```python
from build123d import *

# Parameters (mm, degrees)
SKETCH2_W           = 102
SKETCH2_H           = 50
BOSS_EXTRUDE2_DEPTH = 2
SKETCH1_W           = 98
SKETCH1_H           = 46
BOSS_EXTRUDE1_DEPTH = 2
FILLET1_R           = 2
CUT_EXTRUDE1_DEPTH  = 1.6
CUT_EXTRUDE2_DEPTH  = 4
SKETCH5_OUTSIDE_W   = 126.722
SKETCH5_OUTSIDE_H   = 74.722
SKETCH5_OUTSIDE_W_2 = 95
SKETCH5_OUTSIDE_H_2 = 44
CUT_EXTRUDE3_DEPTH  = 10
SKETCH6_R           = 0.25
CUT_EXTRUDE4_DEPTH  = 10
SKETCH7_R           = 1.7
CUT_EXTRUDE5_DEPTH  = 10


with BuildPart() as part:
    # Sketch2 → Boss-Extrude2 (new body)
    with BuildSketch(Plane(origin=(0, 0, 0), x_dir=(1, 0, 0), z_dir=(0, 1, 0))):
        Rectangle(SKETCH2_W, SKETCH2_H)
    extrude(amount=BOSS_EXTRUDE2_DEPTH)

    # Sketch1 → Boss-Extrude1 (add)
    with BuildSketch(Plane(origin=(0, 0, 0), x_dir=(1, 0, 0), z_dir=(0, 1, 0))):
        Rectangle(SKETCH1_W, SKETCH1_H)
    extrude(amount=BOSS_EXTRUDE1_DEPTH)

    # Fillet1
    fillet1_edges = [part.edges().sort_by_distance(p)[0] for p in [
        (51, 1, 25),
        (-51, 1, 25),
        (-51, 1, -25),
        (51, 1, -25),
    ]]
    fillet(fillet1_edges, radius=FILLET1_R)

    # Sketch3 → Cut-Extrude1 (cut)
    with BuildSketch(Plane(origin=(0, 2, 0), x_dir=(1, 0, 0), z_dir=(0, 1, 0))):
        with BuildLine():
            ThreePointArc((-45.25, 19.75), (-46.957106781, 20.457106781), (-46.25, 18.75))
            Line((-46.25, 18.75), (-46.25, 19.75))
            Line((-46.25, 19.75), (-45.25, 19.75))
        make_face()
        with BuildLine():
            Line((-46.25, 19.75), (-46.25, 18.75))
            ThreePointArc((-46.25, 18.75), (-45.542893219, 19.042893219), (-45.25, 19.75))
            Line((-45.25, 19.75), (-46.25, 19.75))
        make_face()
        with BuildLine():
            Line((-46.25, -18.75), (-46.25, -19.75))
            Line((-46.25, -19.75), (-45.25, -19.75))
            ThreePointArc((-45.25, -19.75), (-45.542893219, -19.042893219), (-46.25, -18.75))
        make_face()
        with BuildLine():
            Line((-45.25, -19.75), (-46.25, -19.75))
            Line((-46.25, -19.75), (-46.25, -18.75))
            ThreePointArc((-46.25, -18.75), (-46.957106781, -20.457106781), (-45.25, -19.75))
        make_face()
        with BuildLine():
            ThreePointArc((46.25, -18.75), (45.542893219, -19.042893219), (45.25, -19.75))
            Line((45.25, -19.75), (46.25, -19.75))
            Line((46.25, -19.75), (46.25, -18.75))
        make_face()
        with BuildLine():
            Line((46.25, -19.75), (45.25, -19.75))
            ThreePointArc((45.25, -19.75), (46.25, -20.75), (47.25, -19.75))
            ThreePointArc((47.25, -19.75), (46.957106781, -19.042893219), (46.25, -18.75))
            Line((46.25, -18.75), (46.25, -19.75))
        make_face()
        with BuildLine():
            ThreePointArc((45.25, 19.75), (45.542893219, 19.042893219), (46.25, 18.75))
            Line((46.25, 18.75), (46.25, 19.75))
            Line((46.25, 19.75), (45.25, 19.75))
        make_face()
        with BuildLine():
            Line((46.25, 19.75), (46.25, 18.75))
            ThreePointArc((46.25, 18.75), (46.957106781, 19.042893219), (47.25, 19.75))
            ThreePointArc((47.25, 19.75), (46.25, 20.75), (45.25, 19.75))
            Line((45.25, 19.75), (46.25, 19.75))
        make_face()
    extrude(amount=-CUT_EXTRUDE1_DEPTH, mode=Mode.SUBTRACT)

    # Sketch4 → Cut-Extrude2 (cut)
    with BuildSketch(Plane(origin=(0, 2, 0), x_dir=(1, 0, 0), z_dir=(0, 1, 0))):
        Polygon((-31, 25), (-31, 21), (-31, 17), (-16, 17), (31, 17), (31, 15), (44, 15), (44, 19), (44, 25), align=None)
    extrude(amount=-CUT_EXTRUDE2_DEPTH, mode=Mode.SUBTRACT)

    # Sketch5 outside → Cut-Extrude3 (cut)
    with BuildSketch(Plane(origin=(0, 2, 0), x_dir=(1, 0, 0), z_dir=(0, 1, 0))):
        Rectangle(SKETCH5_OUTSIDE_W, SKETCH5_OUTSIDE_H)
        Rectangle(SKETCH5_OUTSIDE_W_2, SKETCH5_OUTSIDE_H_2, mode=Mode.SUBTRACT)
    extrude(amount=-CUT_EXTRUDE3_DEPTH, mode=Mode.SUBTRACT)

    # Sketch6 → Cut-Extrude4 (cut)
    with BuildSketch(Plane(origin=(0, 0.4, 0), x_dir=(1, 0, 0), z_dir=(0, 1, 0))):
        with Locations(Location((-46.25, 19.75, 0), (0, 0, 270))):
            Circle(SKETCH6_R)
        with Locations(Location((-46.25, -19.75, 0), (0, 0, 270))):
            Circle(SKETCH6_R)
        with Locations(Location((46.25, 19.75, 0), (0, 0, 270))):
            Circle(SKETCH6_R)
        with Locations(Location((46.25, -19.75, 0), (0, 0, 270))):
            Circle(SKETCH6_R)
    extrude(amount=-CUT_EXTRUDE4_DEPTH, mode=Mode.SUBTRACT)

    # Sketch7 → Cut-Extrude5 (cut)
    with BuildSketch(Plane(origin=(0, 2, 0), x_dir=(1, 0, 0), z_dir=(0, 1, 0))):
        with Locations((-46.25, -19.75)):
            Circle(SKETCH7_R)
        with Locations((-46.25, 19.75)):
            Circle(SKETCH7_R)
        with Locations((46.25, 19.75)):
            Circle(SKETCH7_R)
        with Locations((46.25, -19.75)):
            Circle(SKETCH7_R)
    extrude(amount=-CUT_EXTRUDE5_DEPTH, mode=Mode.SUBTRACT)


solid = part.part
```
Can you work these out from the model? Positions are in its coordinate system, mm. A direction names the side the tool comes from. Round coordinates to 2 decimals unless told otherwise and drop trailing zeros. Order: outer loops, then holes, each group sorted by start corner. A loop starts at its lowest first (then second) coordinate and runs counter-clockwise, first axis right, second up.
(1) If I drill on L1, parallel to Z at x = -46.25, y = 1.3; L2, parallel to Z at x = -11, y = 1.3; L3, parallel to Z at x = 34, y = 1.95, over which ranges is the centre line in solid material (lowest first)?
Results are:
L1: z = -22 to -21.45, -18.05 to 18.05, 21.45 to 22
L2: z = -17 to 22
L3: z = -15 to 22
(2) If we section it at B-B (x = 46.25): Please give me the cut outline in (y, z).
Results are:
outline: (0, -22) - (2, -22) - (2, -21.45) - (0, -21.45) - close; (0, -18.05) - (2, -18.05) - (2, 18.05) - (0, 18.05) - close; (0, 21.45) - (2, 21.45) - (2, 22) - (0, 22) - close
(3) If we section it at D-D (x = 35.5): Please give me the cut outline in (y, z), plus the area to 3 significant figures.
Results are:
outline: (0, -15) - (2, -15) - (2, 22) - (0, 22) - close
area: 74.0 mm2
(4) I'm going to push flat-ended pins straight in: pin 1 (1 mm diameter, centred on x = 35.5, y = 1.5, fed in from -Z); pin 2 (1 mm diameter, centred on x = 7, y = 1.5, fed in from -Z). Where does each tip first touch, or does it pass through?
Results are:
pin 1: stops at z = -15
pin 2: stops at z = -17
(5) If we section it at A-A (z = -16): Please give me the cut outline in (x, y), plus the area to 3 significant figures.
Results are:
outline: (-47.5, 0) - (31, 0) - (31, 2) - (-47.5, 2) - close; (44, 0) - (47.5, 0) - (47.5, 2) - (44, 2) - close
area: 164 mm2
(6) On a 3-axis mill with a long thin cutter (end or side, diameter ignored), from which of +Z, -Z, +X, -X, +Y, -Y can I reach the whole of each face in a straight line? I mean faces 4 (the face through (44.55, 1.01, -19.81)), 5 (the face through (44, 1, -18)). Say none if no direction works.
Results are:
face 4: +Y, -Y
face 5: -Z, +Y, -Y
(7) If we section it at C-C (y = 1.15): Please give me the cut outline in (x, z), plus the area to 3 significant figures.
Results are:
outline: (-47.5, -22) - (-31, -22) - (-31, -17) - (31, -17) - (31, -15) - (44, -15) - (44, -22) - (47.5, -22) - (47.5, -20.9) arc R1.7 cw (long way) to (47.5, -18.6) - (47.5, 18.6) arc R1.7 cw (long way) to (47.5, 20.9) - (47.5, 22) - (-47.5, 22) - (-47.5, 20.9) arc R1.7 cw (long way) to (-47.5, 18.6) - (-47.5, -18.6) arc R1.7 cw (long way) to (-47.5, -20.9) - close
area: 3,750 mm2
(8) We'd pull the mould along X, two halves only. Please class faces 1 (the face through (37, 1, -15)), 2 (the face through (46, 1, -22)), 3 (the face through (47.5, 1, 0)): +X half, -X half, draft (parallel to the pull), parting line (faces both ways), or undercut.
Results are:
face 1: undercut
face 2: draft
face 3: +X half
